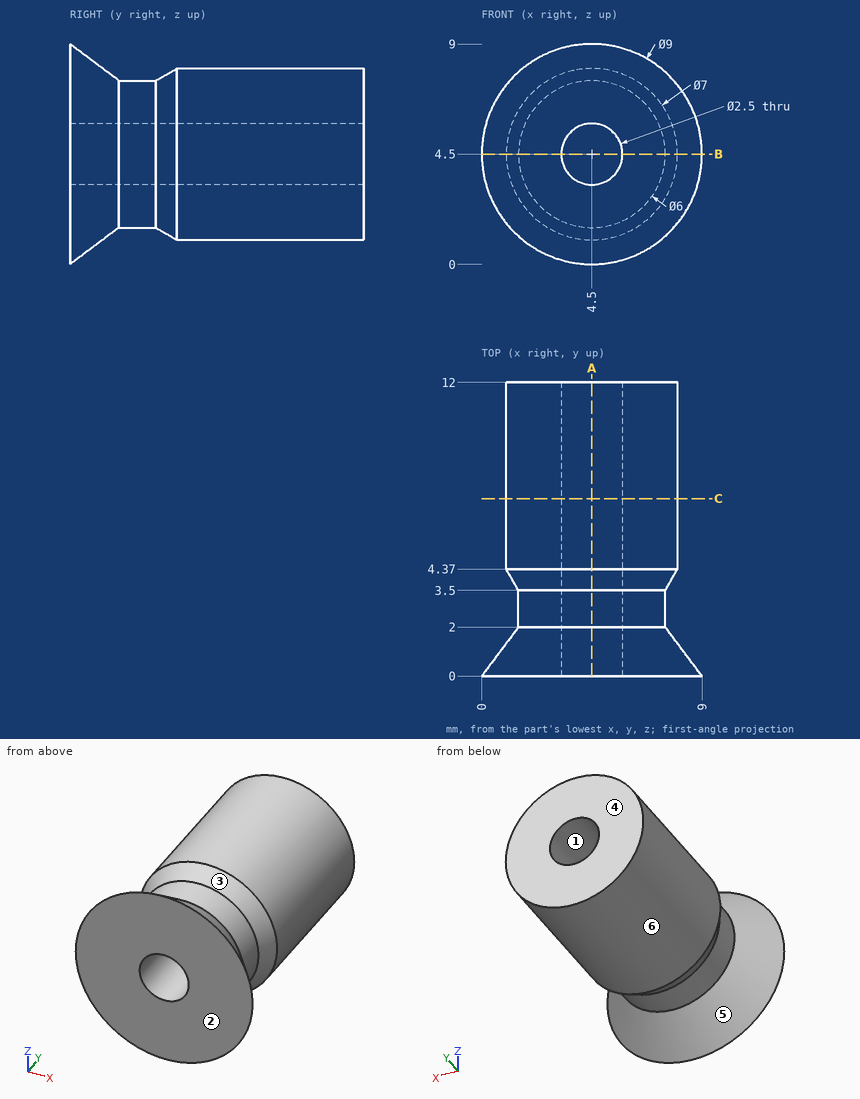
Input: dimensioned drawing with shaded views. Units: mm. Origin: part minimum x, y, z. A direction names the side the tool comes from. Round coordinates to 2 decimals unless told otherwise and drop trailing zeros. Loops run counter-clockwise (first coordinate to the right, second up) from the corner with the lowest first, then second, coordinate; pieces in that order, holes last. Notation, with made-up numbers: M -33,44.5 L -17,44.5 A20 ccw -17,72.5 Z; hole C 28,63 d3. An arc over 180 degrees is marked long. Return JSON: item names as keys, results as strings. Group by question number.
1. Section query C-C on y = 7.25. Output: boundary loops of the cut face in (x, z).
2. Material intervals for line 1 along Z through (x, y) = (4.5, 6.75); line 2 along X through (y, z) = (5.25, 4.25); line 3 along Z through (x, y) = (3.75, 3.5), sorted ascending. Write a range as from..to.
3. Pin query (flat end, axial travel): pin 1 (1 mm diameter, centred on x = 4, y = 10.5, fed in from -Z); pin 2 (2 mm diameter, centred on x = 3, y = 8.5, fed in from +Z); pin 3 (2 mm diameter, centred on x = 4.5, z = 4.5, fed in from +Y); pin 4 (3 mm diameter, centred on x = 7.5, y = 9, fed in from +Z). Return the tip coordinate at first contact, or that it passes through.
4. Reachability of the marked faces 5 and 6 from +Z, -Z, +X, -X, +Y, -Y: full face, straight path, thin tool, end or side. Return the list, or none.
5. Section query B-B on z = 4.5. Output: boundary loops of the cut face in (x, y), and give its area (3 significant figures).
6. Section query A-A on x = 4.5. Output: boundary loops of the cut face in (y, z), and give its area (3 significant figures).
7. Mould query, pull axis Y, two halves, no side actions, for the marked faces 1, 2, 3 and 4. Classes: released by +Y, released by -Y, zero draft, split by the parting line, or undercut.
Checks:
{
 "1": {"outline": "C 4.5,4.5 d7; hole C 4.5,4.5 d2.5"},
 "2": {"line 1": "z = 1..3.25, 5.75..8", "line 2": "x = 1.01..3.28, 5.72..7.99", "line 3": "z = 1.6..3.5, 5.5..7.4"},
 "3": {"pin 1": "stops at z = 1", "pin 2": "stops at z = 7.96", "pin 3": "passes through", "pin 4": "stops at z = 7.66"},
 "4": {"face 5": "none", "face 6": "+Y"},
 "5": {"outline": "M 0,0 L 3.25,0 L 3.25,12 L 1,12 L 1,4.37 L 1.5,3.5 L 1.5,2 Z; M 5.75,0 L 9,0 L 7.5,2 L 7.5,3.5 L 8,4.37 L 8,12 L 5.75,12 Z", "area": "53.1 mm²"},
 "6": {"outline": "M 0,0 L 2,1.5 L 3.5,1.5 L 4.37,1 L 12,1 L 12,3.25 L 0,3.25 Z; M 0,5.75 L 12,5.75 L 12,8 L 4.37,8 L 3.5,7.5 L 2,7.5 L 0,9 Z", "area": "53.1 mm²"},
 "7": {"face 1": "zero draft", "face 2": "released by -Y", "face 3": "undercut", "face 4": "released by +Y"}
}
